Job drawing, mm, ordinate dimensions from the low corner. One solid piece. A direction names the side the tool comes from. Give positions to 0.01 mm unless a question says otherwise; leave off trailing zeros. Order: outer loops, then holes, each group sorted by start corner. A loop starts at its lowest first (then second) coordinate and runs counter-clockwise, first axis right, second up. Notation, with made-up numbers: (69, 70.25) - (86, 70.25) arc R14 cw to (86, 90.25) - close; hole circle Ø1 at (-9.5, -9). An arc over 180 degrees is marked (long way). Use one line per item in the form item = value. Start each with the question number.
1. Band-saw the part on B-B, the plane x = 462. List the corners of the cut face in (y, z), plus the area to 3 significant figures.
2. Tool access for the marked faces 1 and 2: list every direction of +Z, -Z, +X, -X, +Y, -Y with a clear straight run to the whole face (end or side of a thin tool).
3. Drill centre lines: line 1 (Y direction, x = 625, z = 808.5); line 2 (Z direction, x = 1617.5, y = 287); line 3 (Z direction, x = 1204.5, y = 201). Where is each one in solid material? Low to high.
4. Band-saw the part on A-A, the plane y = 155. List the corners of the cut face in (x, z) (1 decimal).
5. Pin check, flat tips, straight feed: P1, Ø8, axis at x = 462.5, z = 324, coming from the +Y side; P2, Ø10, axis at x = 1195, y = 177, coming from the +Z side; P3, Ø5, axis at y = 239.5, z = 606, coming from the +X side. Stop position of each tip, or through.
6. Band-saw the part on D-D, the plane z = 1101. List the corners of the cut face in (x, y).
7. Band-saw the part on C-C, the plane y = 276. List the corners of the cut face in (x, z).
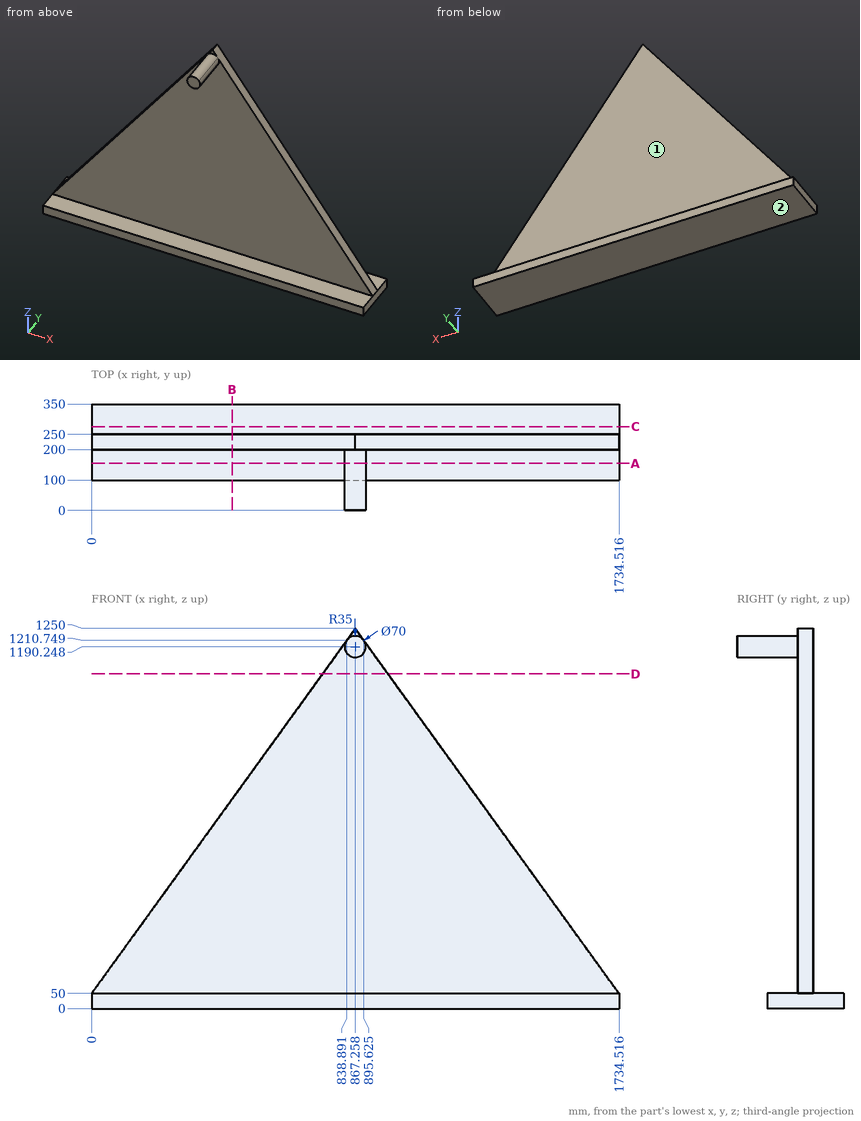
From the geometry:
q1.outline = (100, 0) - (350, 0) - (350, 50) - (250, 50) - (250, 689.26) - (200, 689.26) - (200, 50) - (100, 50) - close
q1.area = 44,500 mm²
q2.face_1 = +Z, +X, -X, +Y
q2.face_2 = -Z, +X, -X, +Y, -Y
q3.line_1 = 200 to 250
q3.line_2 = 0 to 50
q3.line_3 = 0 to 783.37
q4.outline = (0, 0) - (1734.5, 0) - (1734.5, 50) - (0, 50) - close; circle Ø70 at (867.3, 1190.2)
q5.P1 = 250
q5.P2 = 50
q5.P3 = 1334.49
q6.outline = (759.57, 200) - (974.94, 200) - (974.94, 250) - (759.57, 250) - close
q7.outline = (0, 0) - (1734.52, 0) - (1734.52, 50) - (0, 50) - close
